Source: CAD feature listing. Evaluate the final solid. Frame: model axes, mm. Face numbers are marked on the shaded views. A direction names the side the tool comes from. Round coordinates to 2 decimals unless told otherwise and drop trailing zeros. Order: outer loops, then holes, each group sorted by start corner. A loop starts at its lowest first (then second) coordinate and runs counter-clockwise, first axis right, second up.
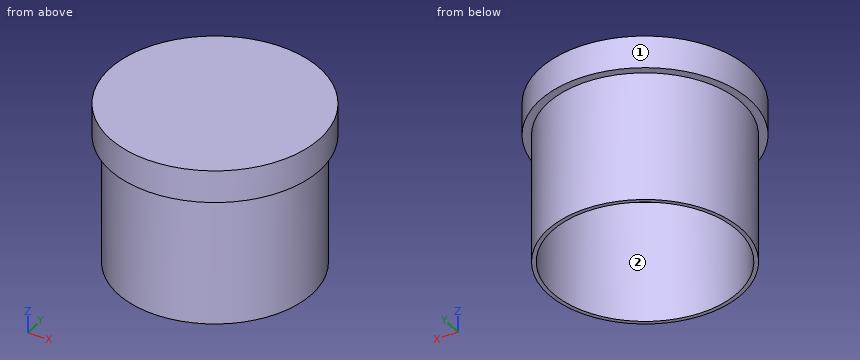
Autodesk Inventor part; units mm, degrees
ref_plane "YZ Plane" through (0, 0, 0) normal (1, 0, 0) x (0, 1, 0)
ref_plane "XZ Plane" through (0, 0, 0) normal (0, 1, 0) x (-1, 0, 0)
ref_plane "XY Plane" through (0, 0, 0) normal (0, 0, 1) x (1, 0, 0)
sketch "Sketch1" plane through (0, 0, 0) normal (0, 0, 1) x (1, 0, 0)
  circle A0 centre (0, 0) radius 76.2
  dimension "tubeDiameter" = 152.4
extrude "Extrusion1" add sketch "Sketch1" along normal mid plane 438.15
sketch "Sketch2" plane through (0, 0, -219.075) normal (0, 0, -1) x (-1, 0, 0)
  circle A0 centre (0, 0) radius 73.025
  dimension "d6" = 146.05
extrude "Extrusion2" cut sketch "Sketch2" against normal blind 406.4
sketch "Sketch3" plane through (0, 0, 219.075) normal (0, 0, 1) x (1, 0, 0)
  circle A0 centre (0, 0) radius 82.55
  circle A1 centre (0, 0) radius 76.2
  dimension "d9" = 165.1
extrude "Extrusion3" add sketch "Sketch3" against normal blind 25.4
sketch "Sketch4" plane through (0, 0, -219.075) normal (0, 0, -1) x (-1, 0, 0)
  circle A0 centre (0, 0) radius 76.2
  circle A1 centre (0, 0) radius 82.55
extrude "Extrusion4" add sketch "Sketch4" against normal blind 25.4
sketch "Sketch7" plane through (0, 0, -219.075) normal (0, 0, -1) x (-1, 0, 0)
  circle A0 centre (0, 0) radius 73.025
  circle A1 centre (0, 0) radius 82.55
  circle A2 centre (0, 0) radius 73.025
  circle A3 centre (0, 0) radius 82.55
extrude "Extrusion6" cut sketch "Sketch7" against normal blind 311.15
properties part number "trussTelescopeTubeRear" material "Aluminum 6061"
1. Line query: line 1 along Y through (x, z) = (0, 165.5) (3 decimals); line 2 along Z through (x, y) = (59, 24) (3 decimals); line 3 along X through (y, z) = (48.5, 156). Output: solid intervals per line, ascending.
2. Section C-C on z = 111.5. Return loops of the section in (x, y) (3 decimals), plus the area to 3 significant figures.
3. Section A-A on x = 0. Return loops of the section in (y, z) (3 decimals), plus the area to 3 significant figures.
4. First-contact query: pin 1 (1.5 mm diameter, centred on x = -23.5, y = 47.5, fed in from -Z) (3 decimals); pin 2 (12 mm diameter, centred on y = -46, z = 116.5, fed in from +X); pin 3 (4 mm diameter, centred on y = 18.5, z = 145.5, fed in from +X). Flat tips, straight axial feed; report the tip coordinate or a pass-through.
5. Access query for the marked faces 1 and 2. Directions: +Z, -Z, +X, -X, +Y, -Y. A direction counts if a zero-diameter tool reaches every point of the face in a straight line with its end or side. Return the directions, or none.
Result:
1. line 1: y = -76.2 to -73.025, 73.025 to 76.2
1. line 2: z = 187.325 to 219.075
1. line 3: x = -58.77 to -54.59, 54.59 to 58.77
2. outline: circle Ø152.4 at (0, 0); hole circle Ø146.05 at (0, 0)
2. area: 1,490 mm2
3. outline: (-82.55, 193.675) - (-76.2, 193.675) - (-76.2, 92.075) - (-73.025, 92.075) - (-73.025, 187.325) - (73.025, 187.325) - (73.025, 92.075) - (76.2, 92.075) - (76.2, 193.675) - (82.55, 193.675) - (82.55, 219.075) - (-82.55, 219.075) - close
3. area: 5,770 mm2
4. pin 1: stops at z = 187.325
4. pin 2: stops at x = 64.86
4. pin 3: stops at x = 74.39
5. face 1: +Z, -Z
5. face 2: -Z
